from build123d import *

# Parameters (mm, degrees)
CYLINDER031_R           = 1.5
CYLINDER031_DEPTH       = 15
CYLINDER031_PITCH_ANGLE = 90
CYLINDER030_R           = 1.5
CYLINDER030_DEPTH       = 15
CYLINDER030_PITCH_ANGLE = 90
SKETCH016_R             = 4.3
EXTRUDE011_DEPTH        = 10
FUSION039_PITCH_ANGLE   = 90


with BuildPart() as m3_hole008:
    # Cylinder031 → Cylinder031 (new body)
    with BuildSketch(Plane.XY):
        Circle(CYLINDER031_R)
    extrude(amount=CYLINDER031_DEPTH)


with BuildPart() as m3_hole008_1:
    # Cylinder031 pitch: moved
    add(m3_hole008.part.rotate(Axis((0, 0, 0), (0, 1, 0)), CYLINDER031_PITCH_ANGLE))


with BuildPart() as m3_hole008_2:
    # Cylinder031 placement: moved
    add(m3_hole008_1.part.moved(Location((163.5, 47, -2.5))))


with BuildPart() as encoder_to_wheel_holes:
    # Cylinder030 → Cylinder030 (new body)
    with BuildSketch(Plane.XY):
        Circle(CYLINDER030_R)
    extrude(amount=CYLINDER030_DEPTH)


with BuildPart() as encoder_to_wheel_holes_1:
    # Cylinder030 pitch: moved
    add(encoder_to_wheel_holes.part.rotate(Axis((0, 0, 0), (0, 1, 0)), CYLINDER030_PITCH_ANGLE))


with BuildPart() as encoder_to_wheel_holes_2:
    # Cylinder030 placement: moved
    add(encoder_to_wheel_holes_1.part.moved(Location((163.5, 47, 22.5))))

    # Fusion096: union M3 hole008
    add(m3_hole008_2.part)


with BuildPart() as extrude011:
    # Sketch016 → Extrude011 (new body)
    with BuildSketch(Plane.XY.offset(2)):
        Circle(SKETCH016_R)
        with BuildLine():
            Line((-1.746425, 2.8), (-1.746425, -2.8))
            ThreePointArc((-1.746425, -2.8), (3.3, 0), (-1.746425, 2.8))
        make_face(mode=Mode.SUBTRACT)
    extrude(amount=EXTRUDE011_DEPTH)


with BuildPart() as encoder_to_wheel_piece:
    # Sketch015 → Revolve (revolve)
    with BuildSketch(Plane.YZ):
        Polygon((18.75, 0), (18.75, 2), (3.75, 2), (1.5, 2), (1.5, 0), (3, 0), align=None)
    revolve(axis=Axis((0, 0, 0), (0, 0, 1)))

    # Fusion039: union Extrude011
    add(extrude011.part)


with BuildPart() as encoder_to_wheel_piece_1:
    # Fusion039 pitch: moved
    add(encoder_to_wheel_piece.part.rotate(Axis((0, 0, 0), (0, 1, 0)), FUSION039_PITCH_ANGLE))


with BuildPart() as encoder_to_wheel_piece_2:
    # Fusion039 placement: moved
    add(encoder_to_wheel_piece_1.part.moved(Location((175, 47, 10))))

    # Cut055: cut Encoder-to-wheel holes
    add(encoder_to_wheel_holes_2.part, mode=Mode.SUBTRACT)


with BuildPart() as encoder_to_wheel_piece_3:
    # Cut055 placement: moved
    add(encoder_to_wheel_piece_2.part.moved(Location((-23, 15, 0))))


with BuildPart() as part_mirroring009:
    # Part__Mirroring009: instance of Encoder-to-wheel piece
    add(encoder_to_wheel_piece_3.part.mirror(Plane(origin=(5, 0, 0), x_dir=(0, -1, 0), z_dir=(1, 0, 0))))


solid = part_mirroring009.part
Work out the finished part from the listing and answer in its coordinate system (mm). A direction names the side the tool comes from. Give positions to 0.01 mm unless a question says otherwise; leave off trailing zeros. Loops run counter-clockwise (first coordinate to the right, second up) from the corner with the lowest first, then second, coordinate; pieces in that order, holes last. Notation, with made-up numbers: (83, 32.25) -> (123, 32.25) arc R16 cw to (123, 62.25) -> close; hole circle Ø8 at (36, -29). An arc over 180 degrees is marked (long way). Use a Markdown table: item, result. Add a question column.
1) Consider line 1 along Z through (x, y) = (-143.4, 62); line 2 along Y through (x, z) = (-150.5, 10); line 3 along X through (y, z) = (56.5, 20.5). Determine where each line is inside the solid, lowest interval first.
2) Which of the six approach directions +Z, -Z, +X, -X, +Y, -Y give full straight-line access (tool end or side, diameter ignored) to faces 4 (the cylindrical face through (-148.9, 61.9, 6.7)), 5 (the flat face through (-154, 62, 12))?
3) Each of these flat-tipped pins is pushed along its axis until it touches: P1, Ø3.5, axis at y = 62, z = 10, coming from the +X side; P2, Ø6, axis at x = -151.5, y = 67.5, coming from the -Z side; P3, Ø1.7, axis at x = -151, y = 63, coming from the -Z side; P4, Ø1.5, axis at x = -148, y = 60.5, coming from the -Z side. Where does it stop, or does it pass through?
4) The part is cut by section A-A, the plane z = 10. Determine the outline of the cut face in (x, y), plus the area to 3 significant figures.
5) For a pull along Y with two mould halves and no side action, classify faces 1 (the flat face through (-149, 62, 11.746)), 2 (the flat face through (-144, 66, 6)), 3 (the cylindrical face through (-148.93, 66.263, 10.56)) as +Y half, -Y half, draft (parallel to the pull), parting line (faces both ways), or undercut.
6) The part is cut by section C-C, the plane x = -151.5. Determine the outline of the cut face in (y, z).
7) The part is cut by section B-B, the plane y = 62. Determine the outline of the cut face in (x, z).
8) The part is cut by section D-D, the plane z = -2.5. Determine the outline of the cut face in (x, y).
Reported:
| question | item | result |
|---|---|---|
| 1 | line 1 | z = -8.75 to -4, -1 to 8.5, 11.5 to 21, 24 to 28.75 |
| 1 | line 2 | y = 57.7 to 58.7, 65.3 to 66.3 |
| 1 | line 3 | x = -144 to -142 |
| 2 | face 4 | -X |
| 2 | face 5 | +Z, -Z, -X, +Y, -Y |
| 3 | P1 | stops at x = -142 |
| 3 | P2 | stops at z = 6.5 |
| 3 | P3 | stops at z = 5.7 |
| 3 | P4 | stops at z = 5.77 |
| 4 | outline | (-154, 57.7) -> (-144, 57.7) -> (-144, 43.25) -> (-142, 43.25) -> (-142, 60.5) -> (-144, 60.5) -> (-144, 58.7) -> (-154, 58.7) -> close; (-154, 65.3) -> (-144, 65.3) -> (-144, 63.5) -> (-142, 63.5) -> (-142, 80.75) -> (-144, 80.75) -> (-144, 66.3) -> (-154, 66.3) -> close |
| 4 | area | 89.0 mm^2 |
| 5 | face 1 | undercut |
| 5 | face 2 | draft |
| 5 | face 3 | parting line |
| 6 | outline | circle Ø8.6 at (62, 10); hole (59.2, 11.75) arc R3.3 ccw (long way) to (64.8, 11.75) -> close |
| 7 | outline | (-154, 5.7) -> (-144, 5.7) -> (-144, -1) -> (-142, -1) -> (-142, 8.5) -> (-144, 8.5) -> (-144, 6.7) -> (-154, 6.7) -> close; (-154, 11.75) -> (-144, 11.75) -> (-144, 11.5) -> (-142, 11.5) -> (-142, 21) -> (-144, 21) -> (-144, 14.3) -> (-154, 14.3) -> close; (-144, -8.75) -> (-142, -8.75) -> (-142, -4) -> (-144, -4) -> close; (-144, 24) -> (-142, 24) -> (-142, 28.75) -> (-144, 28.75) -> close |
| 8 | outline | (-144, 48.02) -> (-142, 48.02) -> (-142, 60.5) -> (-144, 60.5) -> close; (-144, 63.5) -> (-142, 63.5) -> (-142, 75.98) -> (-144, 75.98) -> close |
